Read the model definition and answer for the solid it produces. Units are mm, in the model's axes. Face numbers are marked on the shaded views. A direction names the side the tool comes from. Give positions to 0.01 mm unless a question says otherwise; leave off trailing zeros. Write each loop counter-clockwise with the first axis right and the second up, starting at its lowest first coordinate (ties: lowest second). Pieces come first, ordered by that corner, then holes. Notation, with made-up numbers: (13, 54.5) - (48, 54.5) arc R5 cw to (48, 59.5) - close; hole circle Ø5 at (43, 16). An arc over 180 degrees is marked (long way). Answer as CSV lines item,"result".
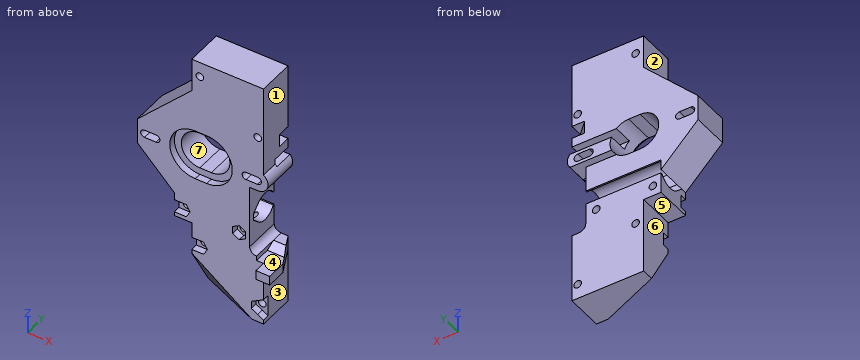
```python
from build123d import *

# Parameters (mm, degrees)
SKETCH001_R     = 1.65
PAD_DEPTH       = 21
POCKET_DEPTH    = 3
POCKET001_DEPTH = 5
POCKET002_DEPTH = 62.9786
SKETCH005_W     = 30
SKETCH005_H     = 3
POCKET003_DEPTH = 8.5
POCKET004_DEPTH = 32.5
POCKET005_DEPTH = 6
POCKET006_DEPTH = 9
POCKET007_DEPTH = 5.5


with BuildPart() as part:
    # Sketch001 → Pad (new body)
    with BuildSketch(Plane.XZ):
        with BuildLine():
            ThreePointArc((21.92031, -4.55), (26.265193, -1.350737), (24.5, 3.748026))
            Line((24.5, 43.5), (24.5, 3.748026))
            Line((-6.5, 43.5), (24.5, 43.5))
            Line((-6.5, 29), (-6.5, 43.5))
            Line((-30, 5.5), (-6.5, 29))
            Line((-30, 5.5), (-30, -5.5))
            Line((-14, -21.5), (-30, -5.5))
            Line((-14, -32), (-14, -21.5))
            Line((-6.5, -32), (-14, -32))
            Line((-6.5, -65), (-6.5, -32))
            Line((24.5, -65), (-6.5, -65))
            Line((24.5, -41), (24.5, -65))
            Line((24.5, -41), (30.5, -41))
            Line((30.5, -41), (30.5, -35))
            Line((21.5, -35), (30.5, -35))
            ThreePointArc((18.5, -32), (19.37868, -34.12132), (21.5, -35))
            Line((18.5, -4.55), (18.5, -32))
            Line((18.5, -4.55), (21.92031, -4.55))
        make_face()
        with Locations((22, 20)):
            Circle(SKETCH001_R, mode=Mode.SUBTRACT)
        with Locations((-3, 37)):
            Circle(SKETCH001_R, mode=Mode.SUBTRACT)
        with Locations((-10.5, -27.5)):
            Circle(SKETCH001_R, mode=Mode.SUBTRACT)
        with Locations((14, -27.5)):
            Circle(SKETCH001_R, mode=Mode.SUBTRACT)
        with Locations((-3, -41.5)):
            Circle(SKETCH001_R, mode=Mode.SUBTRACT)
        with Locations((22, -58.5)):
            Circle(SKETCH001_R, mode=Mode.SUBTRACT)
        with BuildLine():
            ThreePointArc((0, -8), (8, 0), (0, 8))
            Line((0, 8), (-5, 8))
            ThreePointArc((-5, 8), (-13, 0), (-5, -8))
            Line((0, -8), (-5, -8))
        make_face(mode=Mode.SUBTRACT)
        with BuildLine():
            ThreePointArc((16.92031, 1.65), (15.27031, 0), (16.92031, -1.65))
            Line((16.92031, -1.65), (21.92031, -1.65))
            ThreePointArc((21.92031, -1.65), (23.57031, 0), (21.92031, 1.65))
            Line((16.92031, 1.65), (21.92031, 1.65))
        make_face(mode=Mode.SUBTRACT)
        with BuildLine():
            ThreePointArc((-26.92031, 1.65), (-28.57031, 0), (-26.92031, -1.65))
            Line((-26.92031, -1.65), (-21.92031, -1.65))
            ThreePointArc((-21.92031, -1.65), (-20.27031, 0), (-21.92031, 1.65))
            Line((-26.92031, 1.65), (-21.92031, 1.65))
        make_face(mode=Mode.SUBTRACT)
    extrude(amount=PAD_DEPTH)

    # Sketch002 → Pocket (cut)
    with BuildSketch(Plane.XZ.offset(16)):
        Polygon((-8.883419, -24.7), (-12.116581, -24.7), (-14.266838, -24.7), (-14.266838, -30.3), (-12.116581, -30.3), (-8.883419, -30.3), (-7.266838, -27.5), align=None)
        Polygon((14, -24.266838), (11.2, -25.883419), (11.2, -29.116581), (14, -30.733162), (16.8, -29.116581), (16.8, -25.883419), align=None)
        Polygon((22, -55.266838), (19.2, -56.883419), (19.2, -60.116581), (22, -61.733162), (26.2, -64.158033), (26.2, -52.841967), align=None)
        Polygon((-1.383419, -38.7), (-4.616581, -38.7), (-6.766838, -38.7), (-6.766838, -44.3), (-4.616581, -44.3), (-1.383419, -44.3), (0.233162, -41.5), align=None)
        with BuildLine():
            ThreePointArc((0, -11), (11, 0), (0, 11))
            Line((0, 11), (-5, 11))
            ThreePointArc((-5, 11), (-16, 0), (-5, -11))
            Line((0, -11), (-5, -11))
        make_face()
    extrude(amount=-POCKET_DEPTH, mode=Mode.SUBTRACT)

    # Sketch003 → Pocket001 (cut)
    with BuildSketch(Plane.XZ.offset(21)):
        with BuildLine():
            ThreePointArc((21.92031, -4.55), (26.265193, -1.350737), (24.5, 3.748026))
            Line((24.5, 43.5), (24.5, 3.748026))
            Line((-6.5, 43.5), (24.5, 43.5))
            Line((-6.5, 29), (-6.5, 43.5))
            Line((-30, 5.5), (-6.5, 29))
            Line((-30, 5.5), (-30, -5.5))
            Line((-14, -21.5), (-30, -5.5))
            Line((-14, -32), (-14, -21.5))
            Line((-6.5, -32), (-14, -32))
            Line((-6.5, -65), (-6.5, -32))
            Line((24.5, -65), (-6.5, -65))
            Line((24.5, -35), (24.5, -65))
            Line((21.5, -35), (24.5, -35))
            ThreePointArc((18.5, -32), (19.37868, -34.12132), (21.5, -35))
            Line((18.5, -4.55), (18.5, -32))
            Line((18.5, -4.55), (21.92031, -4.55))
        make_face()
    extrude(amount=-POCKET001_DEPTH, mode=Mode.SUBTRACT)

    # Sketch004 → Pocket002 (cut, through all)
    with BuildSketch(Plane(origin=(0, 0, 0), x_dir=(0.590042, 0, 0.807372), z_dir=(-0.807372, 0, 0.590042))):
        Polygon((-56.5, -5), (-56.5, -16), (-41, -16), align=None)
    extrude(amount=-POCKET002_DEPTH, mode=Mode.SUBTRACT)

    # Sketch005 (on Face2 of Pocket002) → Pocket003 (cut)
    with BuildSketch(Plane(origin=(0, 0, 0), x_dir=(1, 0, 0), z_dir=(0, 1, 0))):
        with Locations((15, 4.5)):
            Rectangle(SKETCH005_W, SKETCH005_H)
        with Locations((15, -4.5)):
            Rectangle(SKETCH005_W, SKETCH005_H)
    extrude(amount=-POCKET003_DEPTH, mode=Mode.SUBTRACT)

    # Sketch006 (on Face5 of Pocket003) → Pocket004 (cut)
    with BuildSketch(Plane(origin=(18.5, 0, 0), x_dir=(0, 0, 1), z_dir=(1, 0, 0))):
        with BuildLine():
            ThreePointArc((-24.555141, 10.131972), (-26.069229, 5.006539), (-23, 0.631341))
            Line((-23, 0.631341), (-23, -1))
            Line((-23, -1), (-17, -1))
            Line((-17, -1), (-17, 0.631341))
            ThreePointArc((-17, 0.631341), (-13.930771, 5.006539), (-15.444859, 10.131972))
            Line((-18.5, 13.5), (-15.444859, 10.131972))
            Line((-21.5, 13.5), (-18.5, 13.5))
            Line((-24.555141, 10.131972), (-21.5, 13.5))
        make_face()
    extrude(amount=-POCKET004_DEPTH, mode=Mode.SUBTRACT)

    # Sketch007 (on Face79 of Pocket004) → Pocket005 (cut)
    with BuildSketch(Plane(origin=(0, 0, -41), x_dir=(1, 0, 0), z_dir=(0, 0, -1))):
        Polygon((24.5, 0), (30.5, 12.5), (30.5, 0), align=None)
    extrude(amount=-POCKET005_DEPTH, mode=Mode.SUBTRACT)

    # Sketch008 (on Face78 of Pocket005) → Pocket006 (cut)
    with BuildSketch(Plane(origin=(30.5, 0, 0), x_dir=(0, 0, 1), z_dir=(1, 0, 0))):
        Polygon((-37, 21), (-37, 9), (-35, 5), (-35, 21), align=None)
    extrude(amount=-POCKET006_DEPTH, mode=Mode.SUBTRACT)

    # Sketch009 → Pocket007 (cut)
    with BuildSketch(Plane.XY.offset(10)):
        Polygon((19, 0), (24.5, -5.5), (24.5, 0), align=None)
    extrude(amount=POCKET007_DEPTH, mode=Mode.SUBTRACT)


solid = part.part
```
(1) Find the intervals of material crossed by L1, parallel to Z at x = 14, y = -6; L2, parallel to Z at x = -3, y = -6.25; L3, parallel to X at y = -6.5, z = -27.5, in increasing order.
Worked out:
L1,"z = -65 to -29.15, -13.85 to -6, -3 to 3, 6 to 43.5"
L2,"z = -65 to -43.15, -39.85 to -26.14, -13.86 to -8, 8 to 35.35, 38.65 to 43.5"
L3,"x = -14 to -12.15, -8.85 to 12.35, 15.65 to 18.5"
(2) For the marked faces 1, 2, 3 and 4, determine the directions among +Z, -Z, +X, -X, +Y, -Y from which every point of the face is accessible in a straight line to the end or side of a thin tool.
Worked out:
face 1,"+Z, +X, +Y, -Y"
face 2,"+Z, -X, +Y, -Y"
face 3,"-Z, +X, +Y, -Y"
face 4,"+X, -Y"
(3) A cutting plane is placed at B-B (z = 0). Write down the section's boundary in (x, y), and give its area (3 significant figures).
Worked out:
outline,"(-30, -16) - (-28.57, -16) - (-28.57, 0) - (-30, 0) - close; (-20.27, -16) - (-16, -16) - (-16, -13) - (-13, -13) - (-13, 0) - (-20.27, 0) - close; (8, -13) - (11, -13) - (11, -16) - (15.27, -16) - (15.27, 0) - (8, 0) - close; (23.57, -16) - (26.47, -16) - (26.47, 0) - (23.57, 0) - close"
area,"284 mm^2"
(4) A cutting plane is placed at D-D (y = -2.5). Count the separate pieces of the cut face and the enclosed holes in it, and give its area (3 significant figures).
Worked out:
separate pieces,"3"
enclosed holes,"8"
area,"3,230 mm^2"
(5) Each of these flat-tipped pins is pushed along its axis until it touches: P1, Ø5.5, axis at x = -23.5, y = -7.5, coming from the -Z side; P2, Ø1.2, axis at y = -19, z = -39.5, coming from the -X side; P3, Ø5, axis at x = -11, y = -11, coming from the -Z side. Where does it stop, or does it pass through?
Worked out:
P1,"stops at z = -14.75"
P2,"stops at x = 24.5"
P3,"stops at z = -32"
(6) A cutting plane is placed at A-A (x = 2). Write down the section's boundary in (y, z).
Worked out:
outline,"(-16, -52.24) - (-8.69, -65) - (0, -65) - (0, -23) - (-0.63, -23) arc R6.15 cw to (-10.13, -24.56) - (-13.5, -21.5) - (-13.5, -18.5) - (-10.13, -15.44) arc R6.15 cw to (-0.63, -17) - (0, -17) - (0, -7.75) - (-13, -7.75) - (-13, -10.82) - (-16, -10.82) - close; (-16, 10.82) - (-13, 10.82) - (-13, 7.75) - (0, 7.75) - (0, 43.5) - (-16, 43.5) - close"
(7) The mould has two halves that part along X. Classify the marked faces 5, 6 and 7: +X half, -X half, draft (parallel to the pull), parting line (faces both ways), or undercut.
Worked out:
face 5,"draft"
face 6,"-X half"
face 7,"undercut"
(8) A cutting plane is placed at C-C (z = 20). Write down the section's boundary in (x, y).
Worked out:
outline,"(-15.5, -16) - (20.35, -16) - (20.35, 0) - (-15.5, 0) - close; (23.65, -16) - (24.5, -16) - (24.5, 0) - (23.65, 0) - close"
